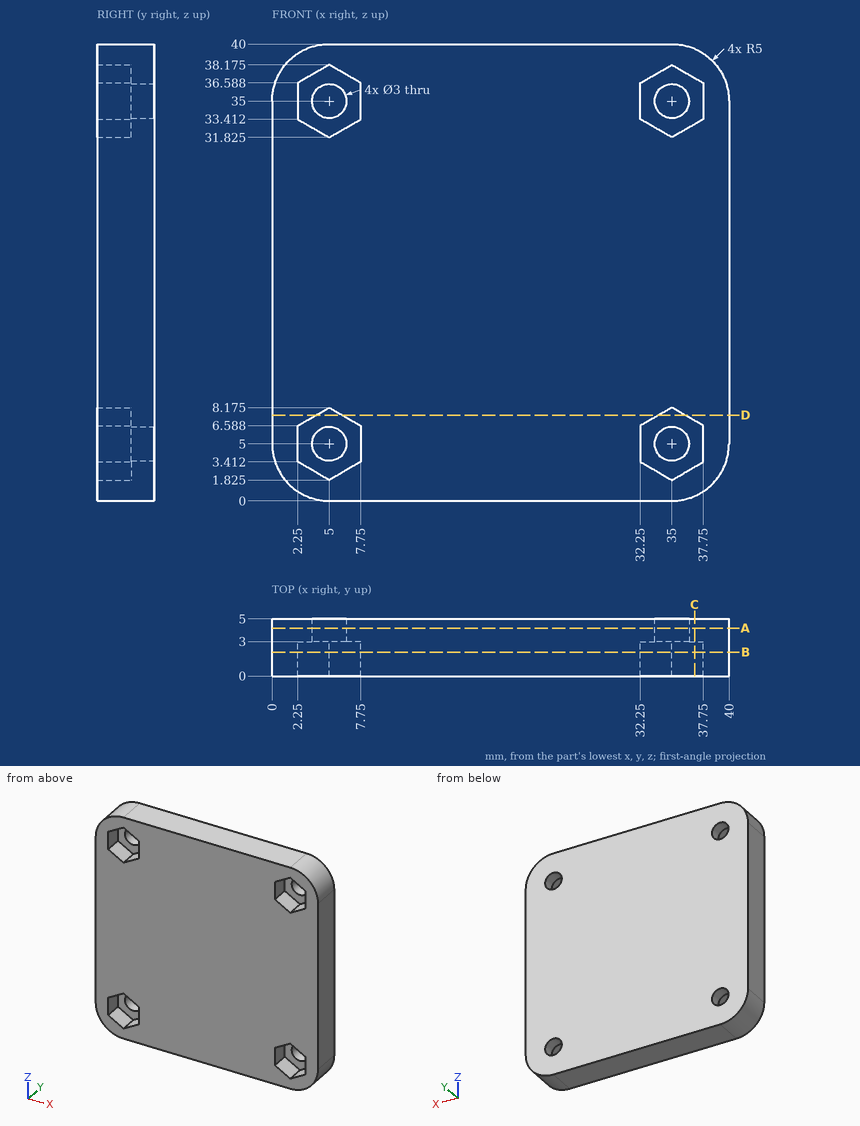
Drawing for the job (mm, zero at the part's lowest x, y, z). Round coordinates to 2 decimals unless told otherwise and drop trailing zeros. Write each loop counter-clockwise with the first axis right and the second up, starting at its lowest first coordinate (ties: lowest second). Pieces come first, ordered by that corner, then holes. Notation, with made-up numbers: M 18.25,78 L 59.25,78 A22 ccw 59.25,87 Z; hole C 55,26.5 d5. An arc over 180 degrees is marked long. Answer in a Markdown table with one row per item.
1. Saw through at C-C (x = 37). List the corners of the cut face in (y, z).
Geometry check:
| item | result |
|---|---|
| outline | M 0,0.42 L 5,0.42 L 5,39.58 L 0,39.58 L 0,37.02 L 3,37.02 L 3,32.98 L 0,32.98 L 0,7.02 L 3,7.02 L 3,2.98 L 0,2.98 Z |
2. Flat gauge pins, fed straight in: P1, Ø3.5, axis at x = 35, z = 5, coming from the -Y side; P2, Ø10, axis at x = 29.5, z = 34.5, coming from the -Y side; P3, Ø1.8, axis at x = 5, z = 35, coming from the +Y side. Where does each tip first touch, or does it go through?
Geometry check:
| item | result |
|---|---|
| P1 | y = 3 |
| P2 | y = 0 |
| P3 | through |
3. Saw through at D-D (z = 7.5). List the corners of the cut face in (x, y).
Geometry check:
| item | result |
|---|---|
| outline | M 0,0 L 3.83,0 L 3.83,3 L 6.17,3 L 6.17,0 L 33.83,0 L 33.83,3 L 36.17,3 L 36.17,0 L 40,0 L 40,5 L 0,5 Z |
4. Saw through at A-A (y = 4.2). List the corners of the cut face in (x, z), and give its area (3 significant figures).
Geometry check:
| item | result |
|---|---|
| outline | M 0,5 A5 ccw 5,0 L 35,0 A5 ccw 40,5 L 40,35 A5 ccw 35,40 L 5,40 A5 ccw 0,35 Z; hole C 5,5 d3; hole C 5,35 d3; hole C 35,5 d3; hole C 35,35 d3 |
| area | 1,550 mm2 |
5. Probe L1, parallel to Z at x = 5, y = 4.45; L2, parallel to X at y = 2.4, z = 6. List the from-to ranges inside material, lowest first. Write a range as [from, to].
Geometry check:
| item | result |
|---|---|
| L1 | [0, 3.5], [6.5, 33.5], [36.5, 40] |
| L2 | [0, 2.25], [7.75, 32.25], [37.75, 40] |
6. Saw through at B-B (y = 2.1). State how many separate pieces and enclosed holes the cut face has, and give its area (3 significant figures).
Geometry check:
| item | result |
|---|---|
| separate pieces | 1 |
| enclosed holes | 4 |
| area | 1,470 mm2 |
